Autodesk Fusion 360 part; units mm, degrees
sketch "Sketch1" plane through (0, 0, 0) normal (0, 0, 1) x (1, 0, 0)
  circle A0 centre (0, 0) radius 10.5
  dimension "d1" = 21
extrude "Extrude1" add sketch "Sketch1" along normal blind 5
sketch "Sketch2" plane through (0, 0, 5) normal (0, 0, 1) x (-1, 0, 0)
  circle A0 centre (0, 0) radius 10.5
  circle A1 centre (0, 0) radius 4
  dimension "d4" = 8
extrude "Extrude2" add sketch "Sketch2" along normal blind 3 contours A1
sketch "Sketch3" plane through (0, 0, 8) normal (0, 0, 1) x (-1, 0, 0)
  circle A0 centre (0, 0) radius 4
  circle A1 centre (0, 0) radius 16
  dimension "d7" = 32
extrude "Extrude3" add sketch "Sketch3" along normal blind 1 contours A0 | A1
sketch "Sketch4" plane through (0, 0, 9) normal (0, 0, 1) x (-1, 0, 0)
  circle A0 centre (0, 0) radius 16
  circle A1 centre (0, 0) radius 7.5
  dimension "d10" = 15
extrude "Extrude4" add sketch "Sketch4" along normal blind 4 contours A1
sketch "Sketch5" plane through (0, 0, 13) normal (0, 0, 1) x (-1, 0, 0)
  circle A0 centre (0, 0) radius 7.5
  circle A1 centre (0, 0) radius 18
  dimension "d13" = 36
extrude "Extrude5" add sketch "Sketch5" along normal blind 19 contours A0 | A1
sketch "Sketch6" plane through (0, 0, 32) normal (0, 0, 1) x (-1, 0, 0)
  circle A0 centre (0, 0) radius 18
  circle A1 centre (0, 0) radius 18.5
  dimension "d16" = 37
extrude "Extrude6" add sketch "Sketch6" along normal blind 34 contours A0 | A1
sketch "Sketch7" plane through (0, 0, 66) normal (0, 0, 1) x (-1, 0, 0)
  circle A0 centre (0, 0) radius 18.5
  circle A1 centre (0, 0) radius 18
  dimension "d19" = 36
extrude "Extrude7" add sketch "Sketch7" along normal blind 4 contours A1
sketch "Sketch8" plane through (0, 0, 70) normal (0, 0, 1) x (-1, 0, 0)
  circle A0 centre (0, 0) radius 18
  circle A1 centre (0, 0) radius 16
  dimension "d22" = 32
extrude "Extrude8" add sketch "Sketch8" along normal blind 28 contours A1
sketch "Sketch9" plane through (0, 0, 98) normal (0, 0, 1) x (-1, 0, 0)
  circle A0 centre (0, 0) radius 16
  line L0 (0, -10) -> (0, 10) construction
  line L1 (9, -4.3589) -> (9, 4.3589)
  line L2 (-9, -4.3589) -> (-9, 4.3589)
  arc A1 (9, 4.3589) -> (-9, 4.3589) centre (0, 0) ccw
  arc A2 (-9, -4.3589) -> (9, -4.3589) centre (0, 0) ccw
  dimension "d25" = 20
  dimension "d26" = 9
sketch "Sketch10" plane through (0, 0, 98) normal (0, 0, 1) x (-1, 0, 0)
extrude "Extrude9" add sketch "Sketch9" along normal blind 3 contours L1 L2 A1 A2
sketch "Sketch11" plane through (0, 0, 101) normal (0, 0, 1) x (-1, 0, 0)
  arc A0 (-9, -4.3589) -> (9, -4.3589) centre (0, 0) ccw
  line L0 (9, -4.3589) -> (9, 4.3589)
  arc A1 (9, 4.3589) -> (-9, 4.3589) centre (0, 0) ccw
  line L1 (-9, 4.3589) -> (-9, -4.3589)
  circle A2 centre (0, 0) radius 3
  dimension "d29" = 6
extrude "Extrude10" add sketch "Sketch11" along normal blind 4 contours A2
sketch "Sketch12" plane through (0, 0, 105) normal (0, 0, 1) x (-1, 0, 0)
  circle A0 centre (0, 0) radius 3
  line L0 (2.7017, -1.3042) -> (2.7017, 1.3042)
  arc A1 (2.7017, 1.3042) -> (2.7017, -1.3042) centre (0, 0) ccw
extrude "Extrude11" add sketch "Sketch12" along normal blind 11 contours A0 L0 A1
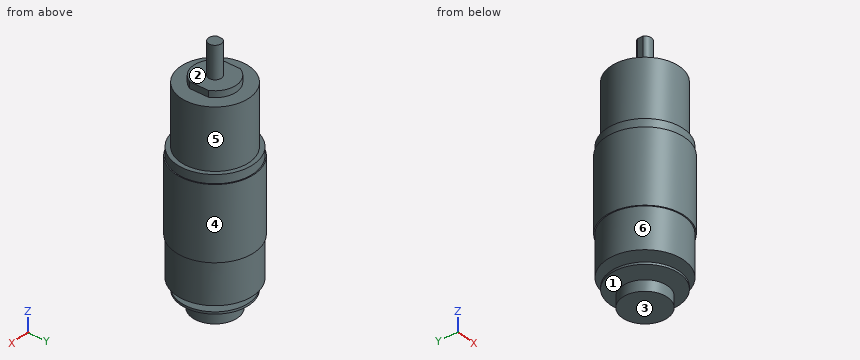
Geometry: final body of the model. Coordinates: model frame, mm. Face numbers are marked on the shaded views. A direction names the side the tool comes from. Coordinates: 2 decimals unless noted, no trailing zeros. Order: outer loops, then holes, each group sorted by start corner. A loop starts at its lowest first (then second) coordinate and runs counter-clockwise, first axis right, second up.
(1) First-contact query: pin 1 (11 mm diameter, centred on x = 8, y = 3.5, fed in from +Z); pin 2 (1.5 mm diameter, centred on y = -1.5, z = 100, fed in from +X); pin 3 (1 mm diameter, centred on y = 6, z = 65, fed in from +X). Flat tips, straight axial feed; report the tip coordinate or a pass-through.
(2) Material intervals for probe 1 along Z at (x, y) = (4.5, 9); probe 2 along Z at (x, y) = (-7, 6.5); probe 3 along Z at (x, y) = (-9.5, -8), sorted ascending.
(3) Access query for the marked faces 4, 5 and 6. Directions: +Z, -Z, +X, -X, +Y, -Y. A direction counts if a zero-diameter tool reaches every point of the face in a straight line with its end or side. Return the directions, or none.
(4) Section query A-A (z = 27). Return the cut outline in (x, y), plus the area to 3 significant figures.
(5) Section query B-B (z = 80.5). Return the cut outline in (x, y).
(6) Draft query along Z for the marked faces 1, 2 and 3. Return one class per face: pulls with the +Z half, pulls with the -Z half, needs draft (parallel to the pull), parting line crosses it, or undercut.
Solution:
1. pin 1: stops at z = 101
1. pin 2: stops at x = 9
1. pin 3: stops at x = 17.66
2. probe 1: z = 0 to 5, 8 to 9, 13 to 98
2. probe 2: z = 0 to 5, 8 to 9, 13 to 101
2. probe 3: z = 8 to 9, 13 to 98
3. face 4: +Z, -Z
3. face 5: +Z
3. face 6: -Z
4. outline: circle Ø36 at (0, 0)
4. area: 1,020 mm2
5. outline: circle Ø32 at (0, 0)
6. face 1: undercut
6. face 2: pulls with the +Z half
6. face 3: pulls with the -Z half
